from build123d import *

# Parameters (mm, degrees)
EXTRUDE_1_DEPTH     = 4
CUT_EXTRUDE_1_DEPTH = 1.5
CUT_EXTRUDE_2_DEPTH = 7.5


with BuildPart() as part:
    # Эскиз1 → Бобышка-Вытянуть1 (new body, symmetric)
    with BuildSketch(Plane.XY):
        Polygon((4, 0), (-4, 0), (-4, -1.5), (-9.75, -1.5), (-9.75, -8), (9.75, -8), (9.75, -1.5), (4, -1.5), align=None)
    extrude(amount=EXTRUDE_1_DEPTH, both=True)

    # Эскиз3 → Отверстие обработанное метчиком M53 (revolve, cut)
    with BuildSketch(Plane(origin=(0, 0, 0), x_dir=(0, 0, 1), z_dir=(1, 0, 0))):
        Polygon((0, 0), (0, 8), (3.1, 8), (2.1, 7), (2.1, 1), (3.1, 0), align=None)
    revolve(axis=Axis((0, 6.35, 0), (0, -1, 0)), mode=Mode.SUBTRACT)

    # Эскиз4 → Вырез-Вытянуть1 (cut)
    with BuildSketch(Plane(origin=(0, 0, 0), x_dir=(1, 0, 0), z_dir=(0, 1, 0))):
        with BuildLine():
            Line((-4, 4), (-4, 0))
            ThreePointArc((-4, 0), (-2.828427125, 2.828427125), (0, 4))
            Line((0, 4), (-4, 4))
        make_face()
        with BuildLine():
            Line((0, -4), (4, -4))
            Line((4, -4), (4, 0))
            ThreePointArc((4, 0), (2.828427125, -2.828427125), (0, -4))
        make_face()
    extrude(amount=-CUT_EXTRUDE_1_DEPTH, mode=Mode.SUBTRACT)

    # Эскиз5 → Вырез-Вытянуть2 (cut, through all)
    with BuildSketch(Plane(origin=(0, -1.5, 0), x_dir=(1, 0, 0), z_dir=(0, 1, 0))):
        with BuildLine():
            Line((-9.75, 0), (-9.75, 4))
            Line((-9.75, 4), (-8.891709622, 4))
            ThreePointArc((-8.891709622, 4), (-9.533012871, 2.045523305), (-9.75, 0))
        make_face()
        with BuildLine():
            Line((9.75, 0), (9.75, -4))
            Line((9.75, -4), (8.891709622, -4))
            ThreePointArc((8.891709622, -4), (9.533012871, -2.045523305), (9.75, 0))
        make_face()
    extrude(amount=-CUT_EXTRUDE_2_DEPTH, mode=Mode.SUBTRACT)

    # Вырез-По траектории1: sweep along a path in Эскиз7
    with BuildLine(Plane.XZ.offset(8)) as sweep_1_path:
        Line((0, 9.75), (-9.75, 9.75))
        Line((-9.75, 9.75), (-9.75, 0))
        ThreePointArc((-9.75, 0), (-6.894291117, -6.894291117), (0, -9.75))
        Line((0, -9.75), (9.75, -9.75))
        Line((9.75, -9.75), (9.75, 0))
        ThreePointArc((9.75, 0), (6.894291117, 6.894291117), (0, 9.75))
    # Эскиз6 → Вырез-По траектории1 (sweep, cut)
    with BuildSketch(Plane.XY.offset(4)):
        Polygon((-9.75, -3), (-9.75, -8), (-4, -8), align=None)
    sweep(path=sweep_1_path.line, transition=Transition.RIGHT, mode=Mode.SUBTRACT)


solid = part.part
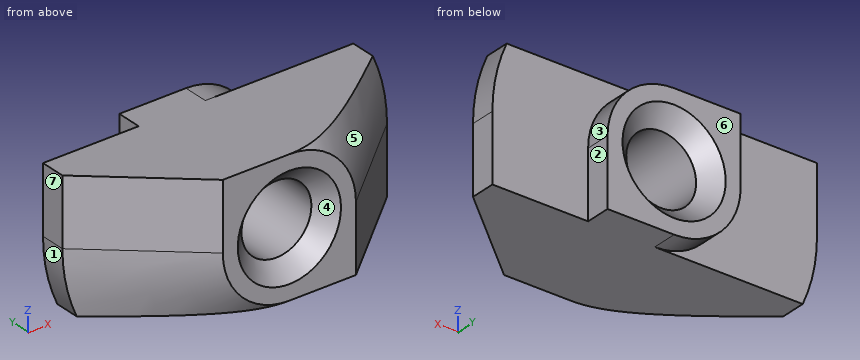
Build history of the part. All positions in model axes, mm. Face numbers are marked on the shaded views. A direction names the side the tool comes from. Give positions to 0.01 mm unless a question says otherwise; leave off trailing zeros. Order: outer loops, then holes, each group sorted by start corner. A loop starts at its lowest first (then second) coordinate and runs counter-clockwise, first axis right, second up. Notation, with made-up numbers: M 56,80 L 73,80 A25 cw 73,102 Z; hole C 24.5,40.5 d3. An arc over 180 degrees is marked long. Use one line per item in the form item = value.
1) Two-plate mould, pull along X, no slides. Class the marked faces 4, 5, 6 and 7: released by +X, released by -X, zero draft, split by the parting line, or undercut.
Calculated:
face_4 = undercut
face_5 = released by +X
face_6 = zero draft
face_7 = released by -X
2) Tool access for the marked faces 1, 2 and 3: list every direction of +Z, -Z, +X, -X, +Y, -Y with a clear straight run to the whole face (end or side of a thin tool).
Calculated:
face_1 = -Z, -X, +Y, -Y
face_2 = +Z, -Z, +X, +Y
face_3 = +Z, +X, +Y
3) Saw through at A-A (y = -2.5). Give the cut face in (x, z), plus the area to 3 significant figures.
Calculated:
outline = M -9.75,0 A9.75 ccw -8.89,-4 L 9.75,-4 L 9.75,0 A9.75 ccw 8.89,4 L -9.75,4 Z; hole C 0,0 d4.2
area = 140 mm2
4) Saw through at B-B (y = -0.25). Give the cut face in (x, z), plus the area to 3 significant figures.
Calculated:
outline = M -4,0 A4 ccw 0,-4 L 4,-4 L 4,0 A4 ccw 0,4 L -4,4 Z; hole C 0,0 d5.7
area = 31.6 mm2
5) Probe probe 1 along Z at (x, y) = (0, -2.7); probe 2 along X at (y, z) = (-2.4, 0); probe 3 along X at (y, z) = (-4.95, 0). List the from-to ranges inside material, lowest first.
Calculated:
probe_1 = -4 to -2.1, 2.1 to 4
probe_2 = -9.75 to -2.1, 2.1 to 9.75
probe_3 = -7.51 to -2.1, 2.1 to 7.51
6) Drop a flat-ended pin along its axis: pin 1 (2 mm diameter, centred on y = -5, z = -1.5, fed in from +X). Give the stop position or say it passes through.
Calculated:
pin_1 = 8.6
